from build123d import *

# Parameters (mm, degrees)
EXTRUDE_1_DEPTH = 15
CHAMFER_1_SIZE  = 1


with BuildPart() as part:
    # 스케치1 → 보스-돌출1 (new body)
    with BuildSketch(Plane.XY):
        Polygon((-8.4, 0), (8.4, 0), (8.4, 3.2), (4.4, 3.2), (4.4, 23.2), (8.2, 23.2), (8.2, 26.4), (-8.2, 26.4), (-8.2, 23.2), (-4.4, 23.2), (-4.4, 3.2), (-8.4, 3.2), align=None)
    extrude(amount=EXTRUDE_1_DEPTH)

    # 모따기1
    chamfer_1_edges = [part.edges().sort_by_distance(p)[0] for p in [
        (4.4, 13.2, 0),
        (0, 0, 0),
        (-4.4, 13.2, 0),
        (0, 26.4, 0),
        (-4.4, 13.2, 15),
        (8.4, 0, 7.5),
        (-8.4, 0, 7.5),
        (-8.2, 26.4, 7.5),
        (8.2, 26.4, 7.5),
        (0, 0, 15),
        (4.4, 13.2, 15),
        (0, 26.4, 15),
    ]]
    chamfer(chamfer_1_edges, length=CHAMFER_1_SIZE)


solid = part.part
Check sheet for the modelled part. Datum: model origin and axes. Units: mm. A direction names the side the tool comes from. Coordinates: 2 decimals unless noted, no trailing zeros. Write each loop counter-clockwise with the first axis right and the second up, starting at its lowest first coordinate (ties: lowest second). Pieces come first, ordered by that corner, then holes.
Item 1: Cross-section at A-A on y = 11.5. Record the boundary of the cut face in (x, z), then the cut area to 3 significant figures.
Numbers:
outline: (-4.4, 1) - (-3.4, 0) - (3.4, 0) - (4.4, 1) - (4.4, 14) - (3.4, 15) - (-3.4, 15) - (-4.4, 14) - close
area: 130 mm2
Item 2: Mould release check, pull along Y, two halves, no side actions. Record for faces 1 (the face through (4.4, 13, 7)), 2 (the face through (6, 3.2, 7)), 3 (the face through (-0.1, 0.5, 14.5)), 4 (the face through (7.7, 25.9, 7.4)): released by +Y, released by -Y, zero draft, split by the parting line, or undercut.
Numbers:
face 1: undercut
face 2: undercut
face 3: released by -Y
face 4: released by +Y
Item 3: Scan lines: probe 1 along Y at (x, z) = (-4.75, 5.5); probe 2 along X at (y, z) = (12.5, 4); probe 3 along Z at (x, y) = (4.25, 21.5). Record each from-to range of solid material in increasing order.
Numbers:
probe 1: y = 0 to 3.2, 23.2 to 26.4
probe 2: x = -4.4 to 4.4
probe 3: z = 0.85 to 14.15
Item 4: Depth check by flat-ended pin: pin 1 Ø4 at (y, z) = (17.5, 11.5) entering from -X; pin 2 Ø1.8 at (y, z) = (25, 4.5) entering from -X; pin 3 Ø4 at (y, z) = (7.5, 9.5) entering from +X. Enter the tip coordinate at first touch or a pass-through.
Numbers:
pin 1: stops at x = -4.4
pin 2: stops at x = -8.2
pin 3: stops at x = 4.4
Item 5: Access from +Z, -Z, +X, -X, +Y, -Y to the whole of each face (thin tool, end or side, straight path). Record for faces 5 (the face through (3.9, 13.1, 0.5)), 6 (the face through (-4.4, 13, 7)), 7 (the face through (-8.2, 24, 7)), 8 (the face through (8.2, 24, 7)), 9 (the face through (-3.9, 13.3, 14.5)).
Numbers:
face 5: -Z, +X
face 6: +Z, -Z, -X
face 7: +Z, -Z, -X, +Y
face 8: +Z, -Z, +X, +Y
face 9: +Z, -X
Item 6: Cross-section at B-B on z = 12.5. Record the boundary of the cut face in (x, y), then the cut area to 3 significant figures.
Numbers:
outline: (-8.4, 1) - (-7.4, 0) - (7.4, 0) - (8.4, 1) - (8.4, 3.2) - (4.4, 3.2) - (4.4, 23.2) - (8.2, 23.2) - (8.2, 25.4) - (7.2, 26.4) - (-7.2, 26.4) - (-8.2, 25.4) - (-8.2, 23.2) - (-4.4, 23.2) - (-4.4, 3.2) - (-8.4, 3.2) - close
area: 280 mm2
